Design review of the part shown in the three views and the two pictorial views. Dimensions are in mm from the part's minimum x, y and z. Give positions to 0.01 mm unless a question says otherwise; leave off trailing zeros. Write each loop counter-clockwise with the first axis right and the second up, starting at its lowest first coordinate (ties: lowest second). Pieces come first, ordered by that corner, then holes.
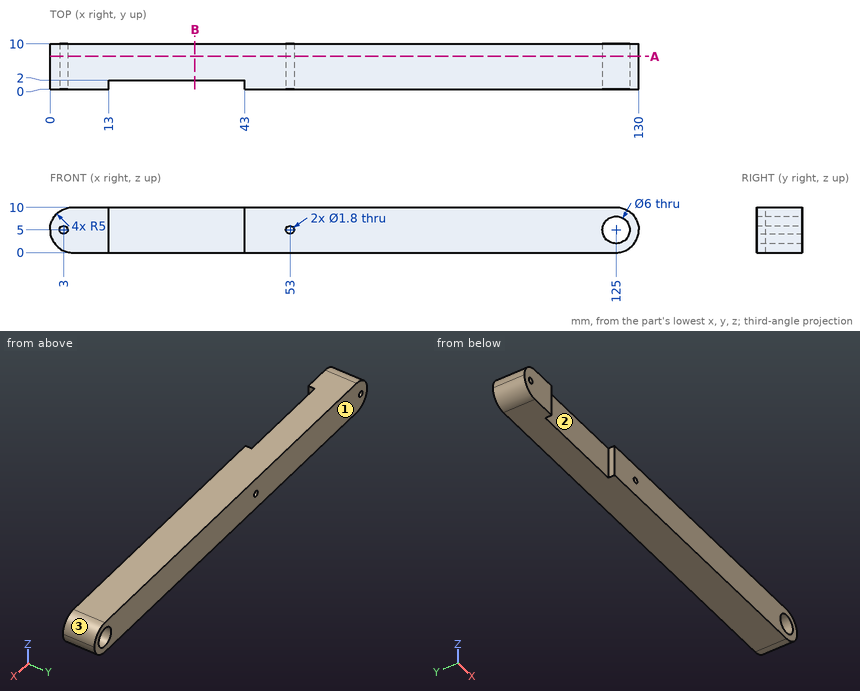
(1) Consider section B-B, the plane x = 32. Give the boundary of the cut face in (y, z), then the cut area to 3 significant figures.
Resolved:
outline: (2, 0) - (10, 0) - (10, 10) - (2, 10) - close
area: 80.0 mm2
(2) To check wall thickness, follow L1, parallel to X at y = 4.75, z = 5; L2, parallel to Z at x = 53, y = 7; L3, parallel to Y at x = 34, z = 3.5. State the ranges of each line that lie inside material, in increasing order.
Resolved:
L1: x = 0 to 2.1, 3.9 to 52.1, 53.9 to 122, 128 to 130
L2: z = 0 to 4.1, 5.9 to 10
L3: y = 2 to 10
(3) Clearance check with flat-ended pins moving along their axes: P1, Ø1.5, axis at x = 86, y = 4, coming from the -Z side; P2, Ø1, axis at y = 7, z = 6, coming from the +X side (3 decimals); P3, Ø5, axis at x = 35, z = 6.5, coming from the -Y side; P4, Ø1.6, axis at y = 1, z = 3, coming from the -X side. State where each tip first meets the part, or that it passes through.
Resolved:
P1: stops at z = 0
P2: stops at x = 129.975
P3: stops at y = 2
P4: stops at x = 0.15
(4) Consider section A-A, the plane y = 7.25. Give the number of separate pieces and of enclosed holes in the cut face, then the cut area to 3 significant figures.
Resolved:
separate pieces: 1
enclosed holes: 3
area: 1,250 mm2
(5) Mouldability with a two-part tool opening along X and no side actions: class the marked faces 1, 2 and 3 as pulls with the +X half, pulls with the -X half, needs draft (parallel to the pull), parting line crosses it, or undercut.
Resolved:
face 1: needs draft
face 2: undercut
face 3: pulls with the +X half
